The model under review builds one solid part; all positions refer to its coordinate system, in mm. A direction names the side the tool comes from. Round coordinates to 2 decimals unless told otherwise and drop trailing zeros. Order: outer loops, then holes, each group sorted by start corner. A loop starts at its lowest first (then second) coordinate and runs counter-clockwise, first axis right, second up.
1) Consider section B-B (y = 108). Give the boundary of the cut face in (x, z).
2) Consider section C-C (z = 5.5). Give the number of separate pieces and of enclosed holes in the cut face, then the cut area to 3 significant figures.
3) Mouldability with a two-part tool opening along Y and no side actions: class faces 3 (the face through (10, 32, 2)), 4 (the face through (22, 0, 3)), 5 (the face through (0, 74, 3)) as pulls with the +Y half, pulls with the -Y half, needs draft (parallel to the pull), parting line crosses it, or undercut.
4) Clearance check with a flat-ended pin moving along its axis: P1, Ø8, axis at x = 23.5, y = 52, coming from the +Z side. State where the tip first meets the part, or that it passes through.
5) Machinability: for faces 1 (the face through (35, 32, 2)), 2 (the face through (22, 61, 3.7)), which of the approach directions +Z, -Z, +X, -X, +Y, -Y give a long, thin tool a straight path to every point of the face, cutting with its end or side? Answer none if there is none.
6) Consider section A-A (x = 26). Give the boundary of the cut face in (y, z).
7) To check wall thickness, follow L1, parallel to Y at x = 18.5, z = 4.5; L2, parallel to Y at x = 10.5, z = 5.5; L3, parallel to X at y = 124.5, z = 5.25. State the ranges of each line that lie inside material, in increasing order.
from build123d import *

# Parameters (mm, degrees)
SKETCH_W     = 45
SKETCH_H     = 150
SKETCH_R     = 1.5
SKETCH_R_2   = 1.6
SKETCH_W_2   = 25
SKETCH_H_2   = 6.75
SKETCH_H_3   = 3
SKETCH_W_3   = 3
SKETCH_H_4   = 20
SKETCH_W_4   = 7.1
SKETCH_H_5   = 7.1
PAD_DEPTH    = 6.7
SKETCH001_W  = 37
SKETCH001_H  = 63
POCKET_DEPTH = 3


with BuildPart() as part:
    # Sketch → Pad (new body)
    with BuildSketch(Plane.XY):
        with Locations((22.5, 75)):
            Rectangle(SKETCH_W, SKETCH_H)
        with Locations((14.933079, 142.899511)):
            Circle(SKETCH_R, mode=Mode.SUBTRACT)
        with Locations((14.933079, 97.399511)):
            Circle(SKETCH_R, mode=Mode.SUBTRACT)
        with Locations((32.433079, 97.399511)):
            Circle(SKETCH_R, mode=Mode.SUBTRACT)
        with Locations((32.433079, 142.899511)):
            Circle(SKETCH_R, mode=Mode.SUBTRACT)
        with Locations((21, 138)):
            Circle(SKETCH_R_2, mode=Mode.SUBTRACT)
        with Locations((30, 108)):
            Circle(SKETCH_R_2, mode=Mode.SUBTRACT)
        with Locations((22.5, 12.052246)):
            Rectangle(SKETCH_W_2, SKETCH_H_2, mode=Mode.SUBTRACT)
        with Locations((22.5, 88.929037)):
            Rectangle(SKETCH_W_2, SKETCH_H_3, mode=Mode.SUBTRACT)
        with Locations((22.5, 31.929037)):
            Rectangle(SKETCH_W_2, SKETCH_H_3, mode=Mode.SUBTRACT)
        with Locations((8.5, 61.019528)):
            Rectangle(SKETCH_W_3, SKETCH_H_4, mode=Mode.SUBTRACT)
        with Locations((36.5, 61.019528)):
            Rectangle(SKETCH_W_3, SKETCH_H_4, mode=Mode.SUBTRACT)
        with Locations((8.55, 126.45)):
            Rectangle(SKETCH_W_4, SKETCH_H_5, mode=Mode.SUBTRACT)
        with Locations((36.65, 126.45)):
            Rectangle(SKETCH_W_4, SKETCH_H_5, mode=Mode.SUBTRACT)
    extrude(amount=PAD_DEPTH)

    # Sketch001 (on Face34 of Pad) → Pocket (cut)
    with BuildSketch(Plane.XY.offset(6.7)):
        with Locations((22.640953, 60.266175)):
            Rectangle(SKETCH001_W, SKETCH001_H)
    extrude(amount=-POCKET_DEPTH, mode=Mode.SUBTRACT)


solid = part.part
Answer below:
1. outline: (0, 0) - (28.4, 0) - (28.4, 6.7) - (0, 6.7) - close; (31.6, 0) - (45, 0) - (45, 6.7) - (31.6, 6.7) - close
2. separate pieces: 1
2. enclosed holes: 10
2. area: 4,110 mm2
3. face 3: undercut
3. face 4: pulls with the -Y half
3. face 5: needs draft
4. P1: stops at z = 3.7
5. face 1: +Z, -Z
5. face 2: +Z
6. outline: (0, 0) - (8.68, 0) - (8.68, 6.7) - (0, 6.7) - close; (15.43, 0) - (30.43, 0) - (30.43, 3.7) - (28.77, 3.7) - (28.77, 6.7) - (15.43, 6.7) - close; (33.43, 0) - (87.43, 0) - (87.43, 3.7) - (33.43, 3.7) - close; (90.43, 0) - (150, 0) - (150, 6.7) - (91.77, 6.7) - (91.77, 3.7) - (90.43, 3.7) - close
7. L1: y = 0 to 8.68, 15.43 to 28.77, 91.77 to 150
7. L2: y = 0 to 8.68, 15.43 to 28.77, 91.77 to 122.9, 130 to 150
7. L3: x = 0 to 5, 12.1 to 33.1, 40.2 to 45
